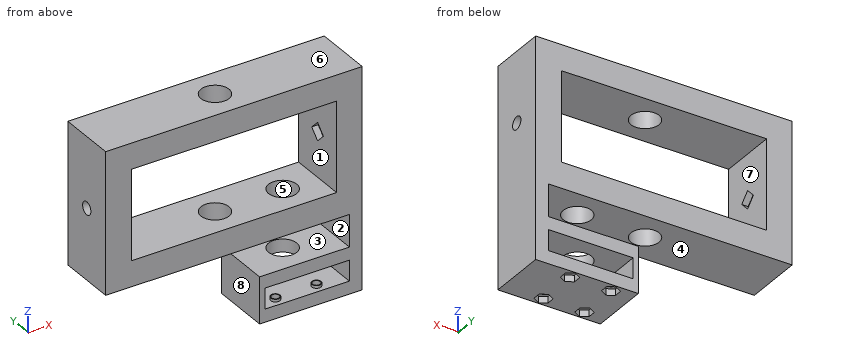
from build123d import *

# Parameters (mm, degrees)
SKETCH1_W           = 100
SKETCH1_H           = 55
SKETCH1_W_2         = 80
SKETCH1_H_2         = 35
BOSS_EXTRUDE1_DEPTH = 11.5
CUT_EXTRUDE1_REACH  = 106.348
SKETCH2_R           = 2.5
CUT_EXTRUDE2_REACH  = 77.215
SKETCH3_R           = 5.5
CUT_EXTRUDE3_START  = -2.5
CUT_EXTRUDE3_DEPTH  = 85
SKETCH5_R           = 5.5
CUT_EXTRUDE4_DEPTH  = 10
SKETCH6_W           = 33
SKETCH6_H           = 8.04
BOSS_EXTRUDE2_DEPTH = 11.5
SKETCH8_R           = 1.8
BOSS_EXTRUDE3_DEPTH = 1
CUT_EXTRUDE5_REACH  = 96.651
SKETCH9_R           = 1.5
CUT_EXTRUDE6_DEPTH  = 2.5
CUT_EXTRUDE7_START  = -5
SKETCH11_R          = 5.5
CUT_EXTRUDE7_DEPTH  = 5


with BuildPart() as part:
    # Sketch1 → Boss-Extrude1 (new, symmetric)
    with BuildSketch(Plane(origin=(0, 0, 0), x_dir=(1, 0, 0), z_dir=(0, 1, 0))):
        Rectangle(SKETCH1_W, SKETCH1_H)
        Rectangle(SKETCH1_W_2, SKETCH1_H_2, mode=Mode.SUBTRACT)
    extrude(amount=BOSS_EXTRUDE1_DEPTH, both=True)

    # Cut-Extrude1: up to this face of the body (flat: up to its plane)
    cut_extrude1_end = Plane(part.part.faces().sort_by_distance((-50, 0, 0))[0])
    # Sketch2 → Cut-Extrude1 (cut, up to the picked face)
    with BuildSketch(Plane(origin=(50, 0, 0), x_dir=(0, 0, -1), z_dir=(1, 0, 0)), mode=Mode.PRIVATE) as cut_extrude1_sk1:
        Circle(SKETCH2_R)
    cut_extrude1_tool1 = split(extrude(cut_extrude1_sk1.sketch, amount=-CUT_EXTRUDE1_REACH, mode=Mode.PRIVATE), bisect_by=cut_extrude1_end, keep=Keep.BOTH, mode=Mode.PRIVATE)
    add(cut_extrude1_tool1.solids().sort_by(Axis((50, 0, 0), (-1, 0, 0)))[0], mode=Mode.SUBTRACT)

    # Cut-Extrude2: up to this face of the body (flat: up to its plane)
    cut_extrude2_end = Plane(part.part.faces().sort_by_distance((0, 0, 27.5))[0])
    # Sketch3 → Cut-Extrude2 (cut, up to the picked face)
    with BuildSketch(Plane(origin=(0, 0, -27.5), x_dir=(-1, 0, 0), z_dir=(0, 0, -1)), mode=Mode.PRIVATE) as cut_extrude2_sk1:
        Circle(SKETCH3_R)
    cut_extrude2_tool1 = split(extrude(cut_extrude2_sk1.sketch, amount=-CUT_EXTRUDE2_REACH, mode=Mode.PRIVATE), bisect_by=cut_extrude2_end, keep=Keep.BOTH, mode=Mode.PRIVATE)
    add(cut_extrude2_tool1.solids().sort_by(Axis((0, 0, -27.5), (0, 0, 1)))[0], mode=Mode.SUBTRACT)

    # Sketch4 → Cut-Extrude3 (cut)
    with BuildSketch(Plane.ZY.offset(-40).offset(CUT_EXTRUDE3_START)):
        with BuildLine():
            ThreePointArc((1.767766953, -1.767766953), (2e-09, -2.5), (-1.767766951, -1.767766955))
            Line((-1.767766951, -1.767766955), (0, -3.535533906))
            Line((0, -3.535533906), (1.767766953, -1.767766953))
        make_face()
        with BuildLine():
            ThreePointArc((-1.767766951, -1.767766955), (-2.5, -2e-09), (-1.767766953, 1.767766953))
            Line((-1.767766953, 1.767766953), (-3.535533906, 0))
            Line((-3.535533906, 0), (-1.767766951, -1.767766955))
        make_face()
        with BuildLine():
            Line((1.767766953, 1.767766953), (0, 3.535533906))
            Line((0, 3.535533906), (-1.767766953, 1.767766953))
            ThreePointArc((-1.767766953, 1.767766953), (0, 2.5), (1.767766953, 1.767766953))
        make_face()
        with BuildLine():
            Line((3.535533906, 0), (1.767766953, 1.767766953))
            ThreePointArc((1.767766953, 1.767766953), (2.309698831, 0.956708581), (2.5, 0))
            ThreePointArc((2.5, 0), (2.309698831, -0.956708581), (1.767766953, -1.767766953))
            Line((1.767766953, -1.767766953), (3.535533906, 0))
        make_face()
    extrude(amount=CUT_EXTRUDE3_DEPTH, mode=Mode.SUBTRACT)

    # Sketch5 → Cut-Extrude4 (cut)
    with BuildSketch(Plane.XY.offset(-27.5)):
        with Locations((26.394, 0)):
            Circle(SKETCH5_R)
    extrude(amount=CUT_EXTRUDE4_DEPTH, mode=Mode.SUBTRACT)

    # Sketch6 → Boss-Extrude2 (add, symmetric)
    with BuildSketch(Plane(origin=(0, 0, 0), x_dir=(1, 0, 0), z_dir=(0, 1, 0))):
        Polygon((10, 58.04), (10, 40), (45, 40), (45, 27.5), (50, 27.5), (50, 58.04), align=None)
        with Locations((28.5, 49.02)):
            Rectangle(SKETCH6_W, SKETCH6_H, mode=Mode.SUBTRACT)
    extrude(amount=BOSS_EXTRUDE2_DEPTH, both=True)

    # Sketch8 → Boss-Extrude3 (add)
    with BuildSketch(Plane.XY.offset(-53.04)):
        with Locations(Location((18.394, 8, 0), (0, 0, 180))):
            Circle(SKETCH8_R)
        with Locations(Location((34.394, 8, 0), (0, 0, 180))):
            Circle(SKETCH8_R)
        with Locations(Location((34.394, -8, 0), (0, 0, 180))):
            Circle(SKETCH8_R)
        with Locations(Location((18.394, -8, 0), (0, 0, 180))):
            Circle(SKETCH8_R)
    extrude(amount=BOSS_EXTRUDE3_DEPTH)

    # Sketch9 → Cut-Extrude5 (cut, up to next)
    with BuildSketch(Plane.XY.offset(-52.04), mode=Mode.PRIVATE) as cut_extrude5_sk1:
        with Locations((18.394, 8)):
            Circle(SKETCH9_R)
    cut_extrude5_tool1 = extrude(cut_extrude5_sk1.sketch, amount=-CUT_EXTRUDE5_REACH, mode=Mode.PRIVATE) & part.part
    # Sketch9 → Cut-Extrude5 (cut, up to next)
    with BuildSketch(Plane.XY.offset(-52.04), mode=Mode.PRIVATE) as cut_extrude5_sk2:
        with Locations((34.394, 8)):
            Circle(SKETCH9_R)
    cut_extrude5_tool2 = extrude(cut_extrude5_sk2.sketch, amount=-CUT_EXTRUDE5_REACH, mode=Mode.PRIVATE) & part.part
    # Sketch9 → Cut-Extrude5 (cut, up to next)
    with BuildSketch(Plane.XY.offset(-52.04), mode=Mode.PRIVATE) as cut_extrude5_sk3:
        with Locations((34.394, -8)):
            Circle(SKETCH9_R)
    cut_extrude5_tool3 = extrude(cut_extrude5_sk3.sketch, amount=-CUT_EXTRUDE5_REACH, mode=Mode.PRIVATE) & part.part
    # Sketch9 → Cut-Extrude5 (cut, up to next)
    with BuildSketch(Plane.XY.offset(-52.04), mode=Mode.PRIVATE) as cut_extrude5_sk4:
        with Locations((18.394, -8)):
            Circle(SKETCH9_R)
    cut_extrude5_tool4 = extrude(cut_extrude5_sk4.sketch, amount=-CUT_EXTRUDE5_REACH, mode=Mode.PRIVATE) & part.part
    add(cut_extrude5_tool1.solids().sort_by_distance((18.394, 8, -52.04))[0], mode=Mode.SUBTRACT)
    add(cut_extrude5_tool2.solids().sort_by_distance((34.394, 8, -52.04))[0], mode=Mode.SUBTRACT)
    add(cut_extrude5_tool3.solids().sort_by_distance((34.394, -8, -52.04))[0], mode=Mode.SUBTRACT)
    add(cut_extrude5_tool4.solids().sort_by_distance((18.394, -8, -52.04))[0], mode=Mode.SUBTRACT)

    # Sketch10 → Cut-Extrude6 (cut)
    with BuildSketch(Plane(origin=(0, 0, -58.04), x_dir=(-1, 0, 0), z_dir=(0, 0, -1))):
        Polygon((-31.644, 6.41228676), (-31.644, 9.58771324), (-34.394, 11.175426481), (-37.144, 9.58771324), (-37.144, 6.41228676), (-34.394, 4.824573519), align=None)
        Polygon((-15.644, 6.41228676), (-15.644, 9.58771324), (-18.394, 11.175426481), (-21.144, 9.58771324), (-21.144, 6.41228676), (-18.394, 4.824573519), align=None)
        Polygon((-15.644, -9.58771324), (-15.644, -6.41228676), (-18.394, -4.824573519), (-21.144, -6.41228676), (-21.144, -9.58771324), (-18.394, -11.175426481), align=None)
        Polygon((-31.644, -9.58771324), (-31.644, -6.41228676), (-34.394, -4.824573519), (-37.144, -6.41228676), (-37.144, -9.58771324), (-34.394, -11.175426481), align=None)
    extrude(amount=-CUT_EXTRUDE6_DEPTH, mode=Mode.SUBTRACT)

    # Sketch11 → Cut-Extrude7 (cut)
    with BuildSketch(Plane.XY.offset(-40).offset(CUT_EXTRUDE7_START)):
        with Locations((26.394, 0)):
            Circle(SKETCH11_R)
    extrude(amount=CUT_EXTRUDE7_DEPTH, mode=Mode.SUBTRACT)


solid = part.part
Geometry check sheet. Reference: the model listing, model coordinates, mm. Face numbers are marked on the shaded views. A direction names the side the tool comes from. Give positions to 0.01 mm unless a question says otherwise; leave off trailing zeros. Write each loop counter-clockwise with the first axis right and the second up, starting at its lowest first coordinate (ties: lowest second). Pieces come first, ordered by that corner, then holes. Notation, with made-up numbers: M -6.5,16.25 L 30.5,16.25 A27 ccw 30.5,50.25 Z; hole C 14,53 d3. An arc over 180 degrees is marked long. One line per question, with ' | ' between items.
1. Cross-section at B-B (x = -28.5). Enter the section's corners in (y, z), plus the area to 3 significant figures.
Ans:
outline: M -11.5,-27.5 L 11.5,-27.5 L 11.5,-17.5 L -11.5,-17.5 Z; M -11.5,17.5 L 11.5,17.5 L 11.5,27.5 L -11.5,27.5 Z | area: 460 mm2
2. Cross-section at C-C (x = 0). Enter the section's corners in (y, z).
Ans:
outline: M -11.5,-27.5 L -5.5,-27.5 L -5.5,-17.5 L -11.5,-17.5 Z; M -11.5,17.5 L -5.5,17.5 L -5.5,27.5 L -11.5,27.5 Z; M 5.5,-27.5 L 11.5,-27.5 L 11.5,-17.5 L 5.5,-17.5 Z; M 5.5,17.5 L 11.5,17.5 L 11.5,27.5 L 5.5,27.5 Z
3. Scan lines: line 1 along Z through (x, y) = (10.5, 8.5); line 2 along Z through (x, y) = (28, -7.5); line 3 along Y through (x, z) = (0, 25.5). Record each from-to range of solid material in increasing order. Write a range as from..to.
Ans:
line 1: -58.04..-40, -27.5..-17.5, 17.5..27.5 | line 2: -58.04..-53.04, -45..-40, -27.5..-17.5, 17.5..27.5 | line 3: -11.5..-5.5, 5.5..11.5
4. Cross-section at A-A (z = -14). Enter the section's corners in (x, y), plus the area to 3 significant figures.
Ans:
outline: M -50,-11.5 L -40,-11.5 L -40,11.5 L -50,11.5 Z; M 40,-11.5 L 50,-11.5 L 50,11.5 L 40,11.5 Z | area: 460 mm2
5. Cross-section at D-D (z = -24). Enter the section's corners in (x, y), plus the area to 3 significant figures.
Ans:
outline: M -50,-11.5 L 50,-11.5 L 50,11.5 L -50,11.5 Z; hole C 0,0 d11; hole C 26.39,0 d11 | area: 2,110 mm2
6. Gauge pin test, flat ends, axial feed: pin 1 (3 mm diameter, centred on y = -8, z = -56, fed in from -X); pin 2 (6 mm diameter, centred on y = 0, z = -33.5, fed in from -X); pin 3 (3 mm diameter, centred on x = 35, y = -8.5, fed in from -Z). Record the tip position at first contact, or that the pin passes through.
Ans:
pin 1: x = 10 | pin 2: x = 45 | pin 3: z = -55.54
7. Mould release check, pull along X, two halves, no side actions. Record for the marked faces 1, 2 and 3: released by +X, released by -X, zero draft, split by the parting line, or undercut.
Ans:
face 1: undercut | face 2: released by -X | face 3: zero draft
8. Set-up check for the marked faces 4, 5, 6, 7 and 8: record each of +Z, -Z, +X, -X, +Y, -Y from which the full face is reachable in a straight line by a thin tool's end or side.
Ans:
face 4: -X, +Y, -Y | face 5: none | face 6: +Z, +X, -X, +Y, -Y | face 7: +Y, -Y | face 8: -Z, -X, +Y, -Y
